Answer from the drawing. Dimensions are ordinates in mm from the lowest x, y and z of the part. A direction names the side the tool comes from. Round coordinates to 2 decimals unless told otherwise and drop trailing zeros. Order: outer loops, then holes, each group sorted by start corner. A loop starts at its lowest first (then second) coordinate and runs counter-clockwise, first axis right, second up. Notation, with made-up numbers: M -12,-7 L 29,-7 A18 ccw 29,5 Z; hole C 69,75 d4. An arc over 180 degrees is marked long. Answer as a JSON object with one key per item and string values. Group by question number.
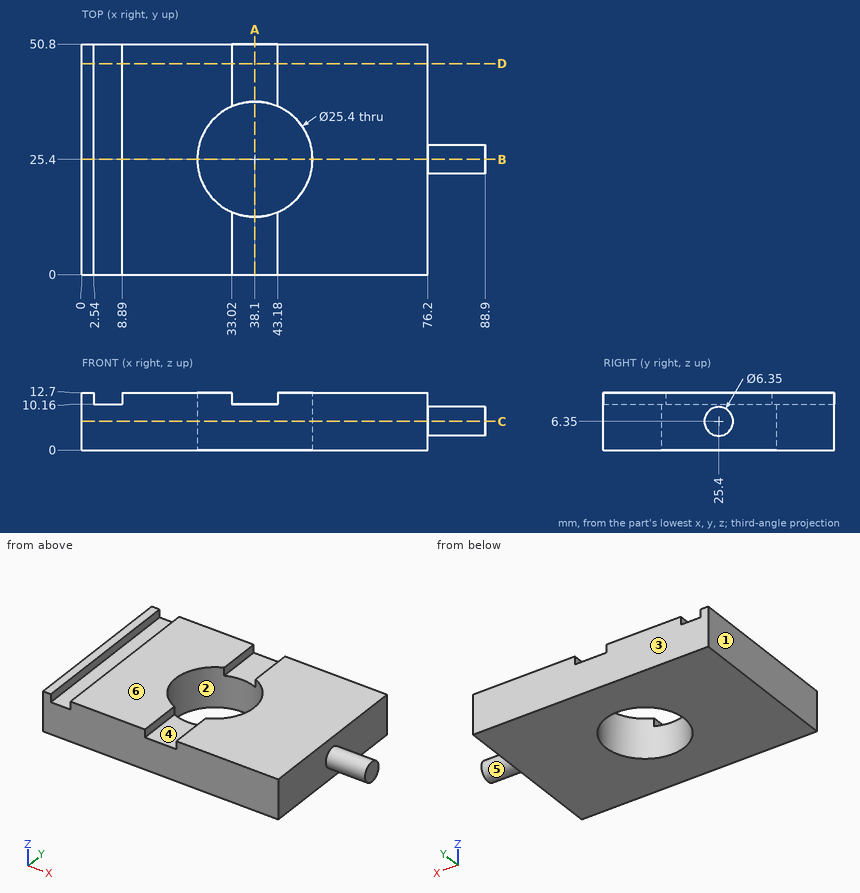
Item 1: Find section D-D (y = 46.5). Give the vertices of the cut face in (x, z).
Item 2: A tool of negligible diameter and unlimited length cuts with its end or side. For the marked faces 4, 5 and 6, from which of +Z, -Z, +X, -X, +Y, -Y can it reach the whole face along a straight path? Write none if from no direction.
Item 3: The mould has two halves that part along X. Classify the marked faces 1, 2 and 3: +X half, -X half, draft (parallel to the pull), parting line (faces both ways), or undercut.
Item 4: Find section C-C (z = 6.35). Give the vertices of the cut face in (x, y) (3 decimals).
Item 5: Each of these flat-tipped pins is pushed along its axis until it touches: pin 1 (5 mm diameter, centred on x = 40, y = 6, fed in from +Z); pin 2 (20.5 mm diameter, centred on x = 38.1, y = 25.4, fed in from -Z); pin 3 (3 mm diameter, centred on y = 34, z = 11, fed in from +X). Where does it stop, or does it pass through?
Item 6: Find section B-B (y = 25.4). Give the vertices of the cut face in (x, z) (3 decimals).
Item 7: Find section A-A (x = 38.1). Give the vertices of the cut face in (y, z), and give its area (3 significant figures).
Item 8: Consider L1, parallel to X at y = 25.4, z = 3.25; L2, parallel to X at y = 27.5, z = 11; L3, parallel to Y at x = 38.1, z = 6.75. Determine where each line is inside the solid, lowest interval first.
Responses:
{
 "1": {"outline": "M 0,0 L 76.2,0 L 76.2,12.7 L 43.18,12.7 L 43.18,10.16 L 33.02,10.16 L 33.02,12.7 L 8.89,12.7 L 8.89,10.16 L 2.54,10.16 L 2.54,12.7 L 0,12.7 Z"},
 "2": {"face 4": "+Z, +Y, -Y", "face 5": "+X", "face 6": "+Z, +X, -X, +Y, -Y"},
 "3": {"face 1": "-X half", "face 2": "undercut", "face 3": "draft"},
 "4": {"outline": "M 0,0 L 76.2,0 L 76.2,22.225 L 88.9,22.225 L 88.9,28.575 L 76.2,28.575 L 76.2,50.8 L 0,50.8 Z; hole C 38.1,25.4 d25.4"},
 "5": {"pin 1": "stops at z = 10.16", "pin 2": "passes through", "pin 3": "stops at x = 76.2"},
 "6": {"outline": "M 0,0 L 25.4,0 L 25.4,12.7 L 8.89,12.7 L 8.89,10.16 L 2.54,10.16 L 2.54,12.7 L 0,12.7 Z; M 50.8,0 L 76.2,0 L 76.2,3.175 L 88.9,3.175 L 88.9,9.525 L 76.2,9.525 L 76.2,12.7 L 50.8,12.7 Z"},
 "7": {"outline": "M 0,0 L 12.7,0 L 12.7,10.16 L 0,10.16 Z; M 38.1,0 L 50.8,0 L 50.8,10.16 L 38.1,10.16 Z", "area": "258 mm^2"},
 "8": {"L1": "x = 0 to 25.4, 50.8 to 88.9", "L2": "x = 0 to 2.54, 8.89 to 25.57, 50.63 to 76.2", "L3": "y = 0 to 12.7, 38.1 to 50.8"}
}
